Geometry check sheet. Reference: the model listing, model coordinates, mm. Face numbers are marked on the shaded views. A direction names the side the tool comes from. Round coordinates to 2 decimals unless told otherwise and drop trailing zeros. Write each loop counter-clockwise with the first axis right and the second up, starting at its lowest first coordinate (ties: lowest second). Pieces come first, ordered by that corner, then holes.
Item 1: Depth check by flat-ended pin: P1, Ø1.5, axis at x = -5, y = -1, coming from the +Z side; P2, Ø1, axis at y = -2.5, z = 12, coming from the +X side; P3, Ø1.5, axis at y = -2, z = 12.5, coming from the +X side. Enter the tip coordinate at first touch or a pass-through.
Item 2: Cross-section at B-B (y = -1.8). Enter the section's corners in (x, z), then the cut area to 3 significant figures.
Item 3: Cross-section at C-C (z = -3.5). Enter the section's corners in (x, y).
Item 4: Draft check along X on the marked faces 1, 2 and 3. Enter one of: pulls with the +X half, pulls with the -X half, needs draft (parallel to the pull), parting line crosses it, or undercut.
Item 5: Cross-section at A-A (z = 6.5). Enter the section's corners in (x, y).
Item 6: Scan lines: probe 1 along X at (y, z) = (-1.3, 6.5); probe 2 along X at (y, z) = (-1.6, 4); probe 3 along Z at (x, y) = (8.5, -1.8). Record each from-to range of solid material in increasing order.
Item 7: Access from +Z, -Z, +X, -X, +Y, -Y to the whole of each face (thin tool, end or side, straight path). Record for the marked faces 4 and 5.
Item 8: Cross-section at D-D (x = 6.5). Enter the section's corners in (y, z).
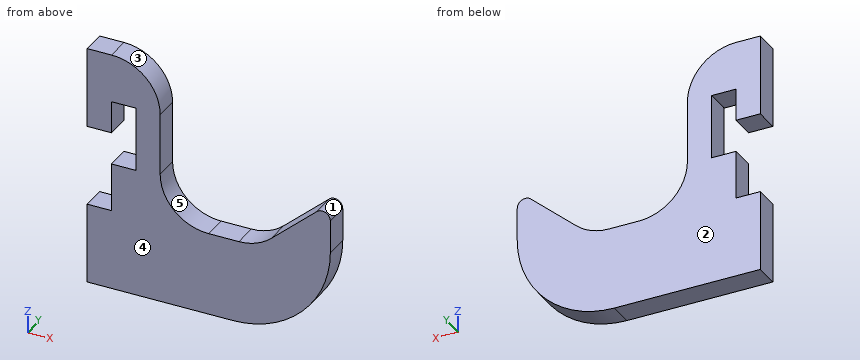
from build123d import *

# Parameters (mm, degrees)
F1_DEPTH = 3


with BuildPart() as f1:
    # F0 (on Front) → F1 (new body)
    with BuildSketch(Plane.XZ):
        with BuildLine():
            Line((-9.316623, -4.437705), (-9.316623, -14.437705))
            Line((-9.316623, -14.437705), (8.688183, -14.437705))
            ThreePointArc((8.688183, -14.437705), (17.173464, -10.922987), (20.688183, -2.437705))
            Line((20.688183, -2.437705), (20.688183, 1.684763))
            ThreePointArc((20.688183, 1.684763), (20.09796, 2.596949), (19.024017, 2.432348))
            Line((19.024017, 2.432348), (13.388086, -2.574695))
            ThreePointArc((13.388086, -2.574695), (11.534632, -3.697795), (9.403091, -4.089183))
            Line((9.403091, -4.089183), (5.683377, -4.089183))
            ThreePointArc((5.683377, -4.089183), (1.440737, -2.331823), (-0.316623, 1.910817))
            Line((-0.316623, 1.910817), (-0.316623, 9.562295))
            ThreePointArc((-0.316623, 9.562295), (-2.073982, 13.804935), (-6.316623, 15.562295))
            Line((-6.316623, 15.562295), (-9.316623, 15.562295))
            Line((-9.316623, 15.562295), (-9.316623, 5.562295))
            Line((-9.316623, 5.562295), (-6.316623, 5.562295))
            Line((-6.316623, 5.562295), (-6.316623, 9.562295))
            Line((-6.316623, 9.562295), (-3.316623, 9.562295))
            Line((-3.316623, 9.562295), (-3.316623, 1.562295))
            Line((-3.316623, 1.562295), (-6.316623, 1.562295))
            Line((-6.316623, 1.562295), (-6.316623, -4.437705))
            Line((-6.316623, -4.437705), (-9.316623, -4.437705))
        make_face()
    extrude(amount=F1_DEPTH)


solid = f1.part
Resolved:
1. P1: stops at z = 15.54
1. P2: stops at x = -0.64
1. P3: stops at x = -0.73
2. outline: (-9.32, -14.44) - (8.69, -14.44) arc R12 ccw to (20.69, -2.44) - (20.69, 1.68) arc R1 ccw to (19.02, 2.43) - (13.39, -2.57) arc R6 cw to (9.4, -4.09) - (5.68, -4.09) arc R6 cw to (-0.32, 1.91) - (-0.32, 9.56) arc R6 ccw to (-6.32, 15.56) - (-9.32, 15.56) - (-9.32, 5.56) - (-6.32, 5.56) - (-6.32, 9.56) - (-3.32, 9.56) - (-3.32, 1.56) - (-6.32, 1.56) - (-6.32, -4.44) - (-9.32, -4.44) - close
2. area: 438 mm2
3. outline: (-6.32, -3) - (3.09, -3) - (3.09, 0) - (-6.32, 0) - close; (12, -3) - (20.64, -3) - (20.64, 0) - (12, 0) - close
4. face 1: undercut
4. face 2: needs draft
4. face 3: pulls with the +X half
5. outline: (-9.32, -3) - (-6.32, -3) - (-6.32, 0) - (-9.32, 0) - close; (-3.32, -3) - (-0.32, -3) - (-0.32, 0) - (-3.32, 0) - close
6. probe 1: x = -9.32 to -6.32, -3.32 to -0.32
6. probe 2: x = -3.32 to -0.32
6. probe 3: z = -14.44 to -4.09
7. face 4: +Z, -Z, +X, -X, -Y
7. face 5: +Z, +Y, -Y
8. outline: (-3, -14.44) - (0, -14.44) - (0, -4.09) - (-3, -4.09) - close
